Verification items for this drawing (mm, ordinates from the low corner). A direction names the side the tool comes from. Round coordinates to 2 decimals unless told otherwise and drop trailing zeros. Write each loop counter-clockwise with the first axis right and the second up, starting at its lowest first coordinate (ties: lowest second). Pieces come first, ordered by that corner, then holes. Notation, with made-up numbers: M 13.25,14 L 20.25,14 A23 cw 20.25,46 Z; hole C -39,66.25 d11. An arc over 180 degrees is marked long. One line per question, with ' | ' between items. Start each with the question number.
Q1. Cross-section at B-B (x = 6.5). Record the boundary of the cut face in (y, z), then the cut area to 3 significant figures.
Q2. Gauge pin test, flat ends, axial feed: pin 1 (1 mm diameter, centred on y = 183, z = 6.5, fed in from -X); pin 2 (10 mm diameter, centred on y = 169, z = 14.5, fed in from -X); pin 3 (3 mm diameter, centred on y = 94.5, z = 3, fed in from -X). Record the tip position at first contact, or that the pin passes through.
Q3. Tool access check on the marked faces 1 and 2. Record the directions out of +Z, -Z, +X, -X, +Y, -Y that give a thin tool (end or side, any length) a straight path to the whole face; none if there is none.
Q4. Thickness scan on line 1 along X through (y, z) = (28, 9.5); line 2 along Y through (x, z) = (13.75, 8.75); line 3 along X through (y, z) = (142.5, 7.5). Record the ranges inside material, lowest first. Write a range as from..to.
Q5. Cross-section at A-A (z = 9). Record the boundary of the cut face in (x, y), then the cut area to 3 significant figures.
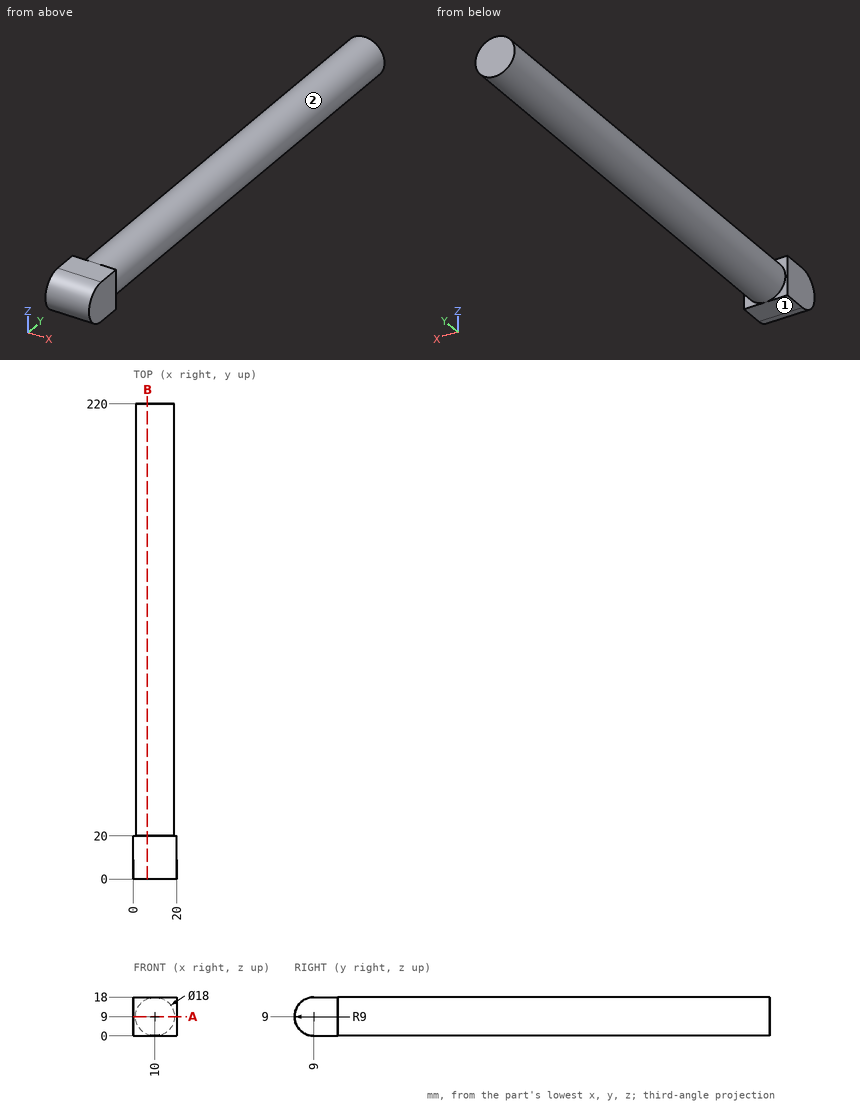
Determined:
1) outline: M 9,0 L 20,0 L 20,0.71 L 220,0.71 L 220,17.29 L 20,17.29 L 20,18 L 9,18 A9 ccw Z | area: 3,640 mm²
2) pin 1: stops at x = 1.23 | pin 2: stops at x = 1.01 | pin 3: stops at x = 2.21
3) face 1: -Z, +X, -X, +Y, -Y | face 2: +Y
4) line 1: x = 1.01..18.99 | line 2: y = 0..220 | line 3: x = 1.13..18.87
5) outline: M 0,0 L 20,0 L 20,20 L 19,20 L 19,220 L 1,220 L 1,20 L 0,20 Z | area: 4,000 mm²
